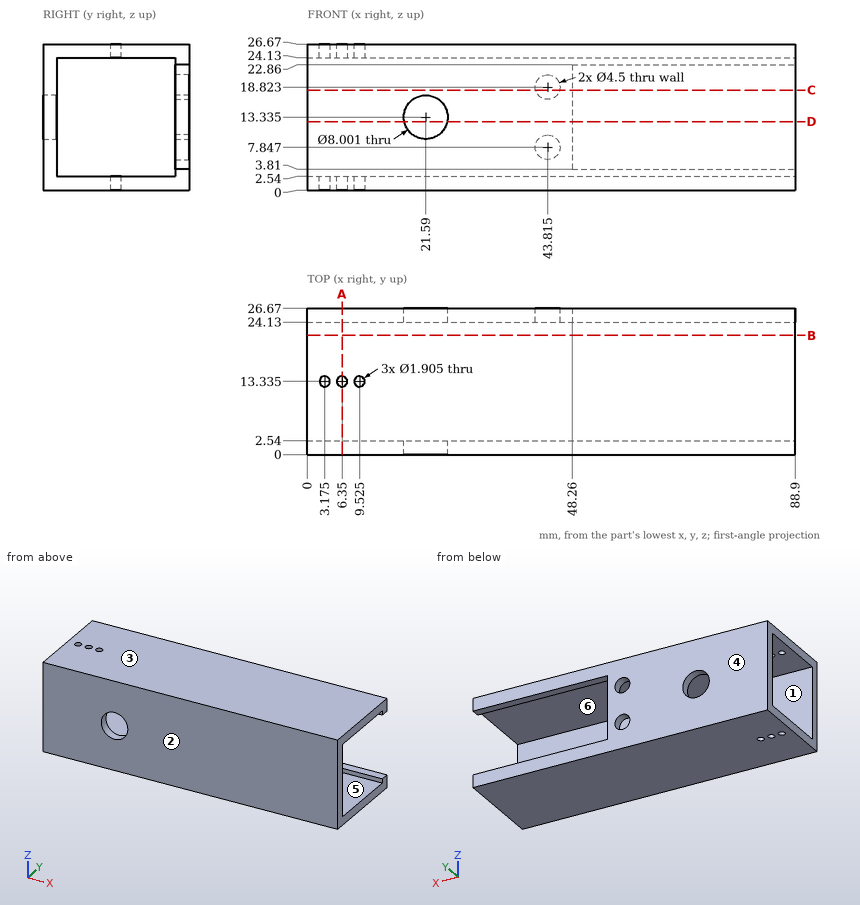
Design review of the part shown in the three views and the two pictorial views. Dimensions are in mm from the part's minimum x, y and z. A direction names the side the tool comes from. Round coordinates to 2 decimals unless told otherwise and drop trailing zeros. Write each loop counter-clockwise with the first axis right and the second up, starting at its lowest first coordinate (ties: lowest second). Pieces come first, ordered by that corner, then holes. Notation, with made-up numbers: (86.25, 22.25) - (129.25, 22.25) arc R16 ccw to (129.25, 38.25) - close; hole circle Ø4 at (39.25, 51.5). An arc over 180 degrees is marked (long way). Answer as CSV lines item,"result". Start each with the question number.
(1) Mouldability with a two-part tool opening along Y and no side actions: class the marked faces 3, 4, 5 and 6 as +Y half, -Y half, draft (parallel to the pull), parting line (faces both ways), or undercut.
(2) Add section B-B, the plane y = 21.75. State the section outline as (x, z) points.
(3) For pin 1 (6 mm diameter, centred on y = 12, z = 4, fed in from +X); pin 2 (3.5 mm diameter, centred on x = 43.82, z = 18.82, fed in from +Y), all flat-tipped, find the tip position at first contact; note any pin that passes through.
(4) Add section A-A, the plane x = 6.35. State the section outline as (y, z) points.
(5) Machinability: for the marked faces 1 and 2, which of the approach directions +Z, -Z, +X, -X, +Y, -Y give a long, thin tool a straight path to every point of the face, cutting with its end or side? Answer none if there is none.
(6) For line 1 (Z direction, x = 83, y = 25.25); line 2 (Y direction, x = 33, z = 7.5), list the stretches that pass through material, from the lowest coordinate up.
(7) Add section D-D, the plane z = 12.5. State the section outline as (x, y) points, plus the area to 3 significant figures.
(8) Add section C-C, the plane z = 18.25. State the section outline as (x, y) points, plus the area to 3 significant figures.
From the geometry:
1,face 3,"draft"
1,face 4,"+Y half"
1,face 5,"undercut"
1,face 6,"undercut"
2,outline,"(0, 0) - (88.9, 0) - (88.9, 2.54) - (0, 2.54) - close; (0, 24.13) - (88.9, 24.13) - (88.9, 26.67) - (0, 26.67) - close"
3,pin 1,"stops at x = 88.9"
3,pin 2,"stops at y = 2.54"
4,outline,"(0, 0) - (12.38, 0) - (12.38, 2.54) - (2.54, 2.54) - (2.54, 24.13) - (12.38, 24.13) - (12.38, 26.67) - (0, 26.67) - close; (14.29, 0) - (26.67, 0) - (26.67, 26.67) - (14.29, 26.67) - (14.29, 24.13) - (24.13, 24.13) - (24.13, 2.54) - (14.29, 2.54) - close"
5,face 1,"+X, -X"
5,face 2,"+Z, -Z, +X, -X, -Y"
6,line 1,"z = 0 to 3.81, 22.86 to 26.67"
6,line 2,"y = 0 to 2.54, 24.13 to 26.67"
7,outline,"(0, 0) - (17.68, 0) - (17.68, 2.54) - (0, 2.54) - close; (0, 24.13) - (17.68, 24.13) - (17.68, 26.67) - (0, 26.67) - close; (25.5, 0) - (88.9, 0) - (88.9, 2.54) - (25.5, 2.54) - close; (25.5, 24.13) - (48.26, 24.13) - (48.26, 26.67) - (25.5, 26.67) - close"
7,area,"309 mm²"
8,outline,"(0, 0) - (88.9, 0) - (88.9, 2.54) - (0, 2.54) - close; (0, 24.13) - (41.64, 24.13) - (41.64, 26.67) - (0, 26.67) - close; (45.99, 24.13) - (48.26, 24.13) - (48.26, 26.67) - (45.99, 26.67) - close"
8,area,"337 mm²"
